```python
from build123d import *

# Parameters (mm, degrees)
SKETCH1_W           = 34
SKETCH1_H           = 60
SKETCH1_R           = 0.75
BOSS_EXTRUDE1_DEPTH = 3
CHAMFER1_SIZE       = 1.3
SKETCH2_R           = 0.762
CUT_EXTRUDE1_DEPTH  = 7
SKETCH3_W           = 5
SKETCH3_H           = 4.4
CUT_EXTRUDE2_DEPTH  = 1.7
SKETCH4_R           = 0.762
CUT_EXTRUDE3_DEPTH  = 7
SKETCH5_W           = 3.3
SKETCH5_H           = 5.3
CUT_EXTRUDE4_DEPTH  = 3.5
SKETCH7_R           = 0.762
SKETCH7_W           = 7
SKETCH7_H           = 5.3
CUT_EXTRUDE5_DEPTH  = 2.5
SKETCH8_W           = 1.8
SKETCH8_H           = 17.3
CUT_EXTRUDE6_DEPTH  = 2.5
SKETCH9_R           = 3.39
CUT_EXTRUDE7_DEPTH  = 7.5


with BuildPart() as part:
    # Sketch1 → Boss-Extrude1 (new body)
    with BuildSketch(Plane.XY):
        Rectangle(SKETCH1_W, SKETCH1_H)
        with Locations((-15, -21.5)):
            Circle(SKETCH1_R, mode=Mode.SUBTRACT)
        with Locations(Location((-10.5, 27.5, 0), (0, 0, 180))):
            Circle(SKETCH1_R, mode=Mode.SUBTRACT)
        with Locations((10.5, 27.5)):
            Circle(SKETCH1_R, mode=Mode.SUBTRACT)
    extrude(amount=BOSS_EXTRUDE1_DEPTH)

    # Chamfer1
    # the kernel refuses this chamfer: 1.3 mm, written as the material it takes off along each edge
    with BuildSketch(Plane(origin=(-15, -21.5, 3), x_dir=(1, 0, 0), z_dir=(0, -1, 0))) as chamfer1_piece_1:
        Polygon((0.75, -CHAMFER1_SIZE), (0.75 + CHAMFER1_SIZE, 0), (0.75, 0), align=None)
    revolve(axis=Axis((-15, -21.5, 3), (0, 0, 1)), mode=Mode.SUBTRACT)
    with BuildSketch(Plane(origin=(-10.5, 27.5, 3), x_dir=(-1, 0, 0), z_dir=(0, 1, 0))) as chamfer1_piece_2:
        Polygon((0.75, -CHAMFER1_SIZE), (0.75 + CHAMFER1_SIZE, 0), (0.75, 0), align=None)
    revolve(axis=Axis((-10.5, 27.5, 3), (0, 0, 1)), mode=Mode.SUBTRACT)
    with BuildSketch(Plane(origin=(10.5, 27.5, 3), x_dir=(1, 0, 0), z_dir=(0, -1, 0))) as chamfer1_piece_3:
        Polygon((0.75, -CHAMFER1_SIZE), (0.75 + CHAMFER1_SIZE, 0), (0.75, 0), align=None)
    revolve(axis=Axis((10.5, 27.5, 3), (0, 0, 1)), mode=Mode.SUBTRACT)

    # Sketch2 → Cut-Extrude1 (cut)
    with BuildSketch(Plane(origin=(17, 0, 0), x_dir=(0, 0, -1), z_dir=(1, 0, 0))):
        with Locations((-1.5, -21.5)):
            Circle(SKETCH2_R)
    extrude(amount=-CUT_EXTRUDE1_DEPTH, mode=Mode.SUBTRACT)

    # Sketch3 → Cut-Extrude2 (cut)
    with BuildSketch(Plane(origin=(0, 0, 0), x_dir=(-1, 0, 0), z_dir=(0, 0, -1))):
        Polygon((3.765333438, -30), (12, -30), (12, -24.8), (7, -24.8), (3.765333438, -24.8), align=None)
        with Locations((9.5, -22.6)):
            Rectangle(SKETCH3_W, SKETCH3_H)
    extrude(amount=-CUT_EXTRUDE2_DEPTH, mode=Mode.SUBTRACT)

    # Sketch4 → Cut-Extrude3 (cut)
    with BuildSketch(Plane.XZ.offset(30)):
        with Locations(Location((15, 1.5, 0), (0, 0, 270))):
            Circle(SKETCH4_R)
    extrude(amount=-CUT_EXTRUDE3_DEPTH, mode=Mode.SUBTRACT)

    # Sketch5 → Cut-Extrude4 (cut)
    with BuildSketch(Plane(origin=(0, 0, 0), x_dir=(-1, 0, 0), z_dir=(0, 0, -1))):
        with Locations((0, 3.425)):
            Rectangle(SKETCH5_W, SKETCH5_H)
    extrude(amount=-CUT_EXTRUDE4_DEPTH, mode=Mode.SUBTRACT)

    # Sketch7 → Cut-Extrude5 (cut)
    with BuildSketch(Plane(origin=(0, 0, 0), x_dir=(-1, 0, 0), z_dir=(0, 0, -1))):
        with Locations((-10.25, 13.75)):
            Circle(SKETCH7_R)
        with Locations((10.25, 13.75)):
            Circle(SKETCH7_R)
        with Locations(Location((10.25, -6.9, 0), (0, 0, 180))):
            Circle(SKETCH7_R)
        with Locations(Location((-10.25, -6.9, 0), (0, 0, 180))):
            Circle(SKETCH7_R)
        with Locations((0, 13.2)):
            Rectangle(SKETCH7_W, SKETCH7_H)
        with Locations((0, -6.35)):
            Rectangle(SKETCH7_W, SKETCH7_H)
    extrude(amount=-CUT_EXTRUDE5_DEPTH, mode=Mode.SUBTRACT)

    # Sketch8 → Cut-Extrude6 (cut)
    with BuildSketch(Plane(origin=(0, 0, 0), x_dir=(-1, 0, 0), z_dir=(0, 0, -1))):
        with Locations((11.8, 3.53)):
            Rectangle(SKETCH8_W, SKETCH8_H)
        with Locations((-11.8, 3.53)):
            Rectangle(SKETCH8_W, SKETCH8_H)
    extrude(amount=-CUT_EXTRUDE6_DEPTH, mode=Mode.SUBTRACT)

    # Sketch9 → Cut-Extrude7 (cut)
    with BuildSketch(Plane(origin=(0, 0, 0), x_dir=(-1, 0, 0), z_dir=(0, 0, -1))):
        with Locations((-1, -15.04)):
            Circle(SKETCH9_R)
    extrude(amount=-CUT_EXTRUDE7_DEPTH, mode=Mode.SUBTRACT)


solid = part.part
```
Verification items for the finished model (mm, model axes). A direction names the side the tool comes from. Coordinates: 2 decimals unless noted, no trailing zeros. Loops run counter-clockwise (first coordinate to the right, second up) from the corner with the lowest first, then second, coordinate; pieces in that order, holes last. Notation, with made-up numbers: (74.5, 74) -> (108.5, 74) arc R21 ccw to (108.5, 110) -> close; hole circle Ø5 at (83.5, -37.75). An arc over 180 degrees is marked (long way). Answer in a Markdown table with one row per item. Add a question column.
1. Section check B-B, the plane x = 1. Enter the section's corners in (y, z) (3 decimals).
2. Draft check along Y on faces 6 (the face through (0, 0, 3)), 7 (the face through (-11.01, -6.93, 1.23)), 8 (the face through (0, -30, 1)). Enter one of: +Y half, -Y half, draft (parallel to the pull), parting line (faces both ways), or undercut.
3. Section check D-D, the plane y = 1.5. Enter the section's corners in (x, z), then the cut area to 3 significant figures.
4. Section check A-A, the plane y = -15.04. Enter the section's corners in (x, z).
5. Section check C-C, the plane y = 7.5. Enter the section's corners in (x, z), then the cut area to 3 significant figures.
6. Access from +Z, -Z, +X, -X, +Y, -Y to the whole of each face (thin tool, end or side, straight path). Record for faces 1 (the face through (-10, -7, 2.5)), 2 (the face through (-17, 0, 1)), 3 (the face through (-12, -25, 1)), 4 (the face through (-1.65, 3, 1)), 5 (the face through (15, -23, 2)).
7. Depth check by flat-ended pin: P1, Ø1.4, axis at x = 15, z = 1.5, coming from the -Y side; P2, Ø1.2, axis at y = -21.5, z = 1.5, coming from the +X side; P3, Ø0.5, axis at x = -10, z = 1, coming from the -Y side. Enter the tip coordinate at first touch or a pass-through.
8. Material ranges on probe 1 along X at (y, z) = (9.5, 2.15); probe 2 along X at (y, z) = (5, 2.3); probe 3 along Y at (x, z) = (12, 1.5), recorded low to high. Write a range as [from, to].
Derived:
| question | item | result |
|---|---|---|
| 1 | outline | (-30, 0) -> (-18.43, 0) -> (-18.43, 3) -> (-30, 3) -> close; (-11.65, 0) -> (-9, 0) -> (-9, 2.5) -> (-3.7, 2.5) -> (-3.7, 0) -> (0.775, 0) -> (0.775, 3) -> (-11.65, 3) -> close; (6.075, 0) -> (10.55, 0) -> (10.55, 2.5) -> (15.85, 2.5) -> (15.85, 0) -> (30, 0) -> (30, 3) -> (6.075, 3) -> close |
| 2 | face 6 | draft |
| 2 | face 7 | undercut |
| 2 | face 8 | -Y half |
| 3 | outline | (-17, 0) -> (-12.7, 0) -> (-12.7, 2.5) -> (-10.9, 2.5) -> (-10.9, 0) -> (-1.65, 0) -> (-1.65, 3) -> (-17, 3) -> close; (1.65, 0) -> (10.9, 0) -> (10.9, 2.5) -> (12.7, 2.5) -> (12.7, 0) -> (17, 0) -> (17, 3) -> (1.65, 3) -> close |
| 3 | area | 83.1 mm² |
| 4 | outline | (-17, 0) -> (-2.39, 0) -> (-2.39, 3) -> (-17, 3) -> close; (4.39, 0) -> (17, 0) -> (17, 3) -> (4.39, 3) -> close |
| 5 | outline | (-17, 0) -> (-12.7, 0) -> (-12.7, 2.5) -> (-10.9, 2.5) -> (-10.9, 0) -> (10.9, 0) -> (10.9, 2.5) -> (12.7, 2.5) -> (12.7, 0) -> (17, 0) -> (17, 3) -> (-17, 3) -> close |
| 5 | area | 93.0 mm² |
| 6 | face 1 | -Z |
| 6 | face 2 | +Z, -Z, -X, +Y, -Y |
| 6 | face 3 | -Z, -Y |
| 6 | face 4 | +Z, -Z |
| 6 | face 5 | -Y |
| 7 | P1 | stops at y = -23 |
| 7 | P2 | stops at x = 10 |
| 7 | P3 | stops at y = -20.4 |
| 8 | probe 1 | x = [-17, -12.7], [-10.9, 10.9], [12.7, 17] |
| 8 | probe 2 | x = [-17, -12.7], [-10.9, -1.65], [1.65, 10.9], [12.7, 17] |
| 8 | probe 3 | y = [-30, -22.26], [-20.74, -5.12], [12.18, 30] |
